Geometry: final body of the model. Coordinates: model frame, mm. Face numbers are marked on the shaded views. Round coordinates to 2 decimals unless told otherwise and drop trailing zeros. Loops run counter-clockwise (first coordinate to the right, second up) from the corner with the lowest first, then second, coordinate; pieces in that order, holes last. Notation, with made-up numbers: M 78.5,-30.75 L 105.5,-30.75 A34 ccw 105.5,8.25 Z; hole C 66,-3.75 d11. An arc over 180 degrees is marked long. Return JSON: item names as keys, results as strings.
from build123d import *

# Parameters (mm, degrees)
F0_W        = 1070
F0_H        = 200
F1_DEPTH    = 80
F2_T        = 8
F3_T1_DEPTH = 1070
F4_D        = 60
F5_D        = 15


# Not quite as in the source:
# - a fillet or chamfer that OpenCascade refuses, or shapes differently, is made with other operations: its cross-section is extruded or revolved along the edge and cut away or added


with BuildPart() as f1:
    # F0 (on Front) → F1 (new body)
    with BuildSketch(Plane.XZ):
        Rectangle(F0_W, F0_H)
    extrude(amount=-F1_DEPTH)

    # F2
    f2_openings = [f1.faces().sort_by_distance(p)[0] for p in [
        (0, 80, 0),
        (535, 40, 0),
        (-535, 40, 0),
    ]]
    offset(amount=F2_T, openings=f2_openings, kind=Kind.INTERSECTION)

    # F3: fillet of radius 10 on 2 edges, made by hand

    # F3_s2 → F3_t1 (join)
    with BuildSketch(Plane.YZ.offset(-535)):
        with BuildLine():
            ThreePointArc((10, -100), (2.9289321881, -97.0710678119), (0, -90))
            Line((0, -90), (0, -100))
            Line((0, -100), (10, -100))
        make_face()
        with BuildLine():
            ThreePointArc((0, 90), (2.9289321881, 97.0710678119), (10, 100))
            Line((10, 100), (0, 100))
            Line((0, 100), (0, 90))
        make_face()
    extrude(amount=F3_T1_DEPTH)

    # F4 (through all)
    with Locations(Plane(origin=(0, 0, 0), x_dir=(1, 0, 0), z_dir=(0, 1, 0))):
        with Locations((0, 0)):
            Hole(F4_D / 2)

    # F5 (through all)
    with Locations(Plane(origin=(0, 0, 0), x_dir=(1, 0, 0), z_dir=(0, 1, 0))):
        with Locations((-51, -51), (51, -51), (51, 51), (-51, 51)):
            Hole(F5_D / 2)


solid = f1.part
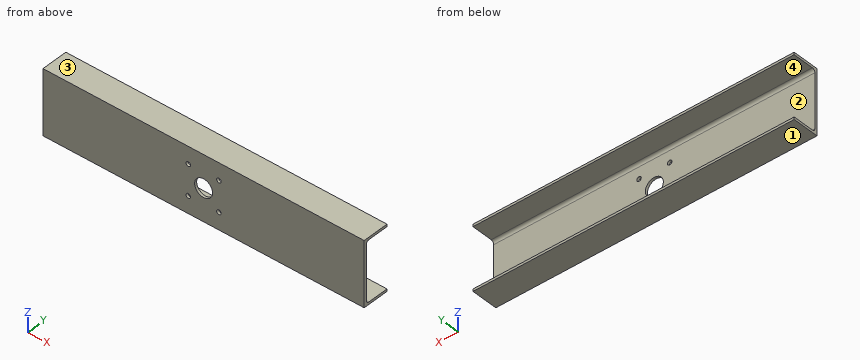
Q1. Section query A-A (x = 0). Output: boundary loops of the cut face in (y, z), plus the area to 3 significant figures.
Determined:
{"outline": "M -8,-108 L 80,-108 L 80,-100 L 10,-100 A10 cw 0,-90 L 0,-30 L -8,-30 Z; M -8,30 L 0,30 L 0,90 A10 cw 10,100 L 80,100 L 80,108 L -8,108 Z", "area": "2,570 mm^2"}
Q2. Material intervals for L1, parallel to Z at x = 51, y = -4.5; L2, parallel to X at y = -1.75, z = -51; L3, parallel to Z at x = 1.5, y = 9.5, sorted ascending.
Determined:
{"L1": "z = -108 to -58.5, -43.5 to 43.5, 58.5 to 108", "L2": "x = -535 to -58.5, -43.5 to 43.5, 58.5 to 535", "L3": "z = -108 to -99.99, 99.99 to 108"}
Q3. Section query B-B (z = 0). Output: boundary loops of the cut face in (x, y).
Determined:
{"outline": "M -535,-8 L -30,-8 L -30,0 L -535,0 Z; M 30,-8 L 535,-8 L 535,0 L 30,0 Z"}
Q4. Pull-direction query (Z, two-part tool) for the marked faces 1, 2, 3 and 4; classes: pulls with the +Z half, pulls with the -Z half, needs draft (parallel to the pull), parting line crosses it, or undercut.
Determined:
{"face 1": "pulls with the -Z half", "face 2": "undercut", "face 3": "pulls with the +Z half", "face 4": "undercut"}
Q5. Section query D-D (x = -312.5). Output: boundary loops of the cut face in (y, z).
Determined:
{"outline": "M -8,-108 L 80,-108 L 80,-100 L 10,-100 A10 cw 0,-90 L 0,90 A10 cw 10,100 L 80,100 L 80,108 L -8,108 Z"}
Q6. Section query C-C (y = 32.5). Output: boundary loops of the cut face in (x, z).
Determined:
{"outline": "M -535,-108 L 535,-108 L 535,-100 L -535,-100 Z; M -535,100 L 535,100 L 535,108 L -535,108 Z"}
